```python
from build123d import *

# Parameters (mm, degrees)
FLOOR_2_DEPTH       = 5
SKETCH2_R           = 1.25
BOSS_EXTRUDE1_DEPTH = 5


with BuildPart() as part:
    # Sketch1 → Floor 2 (new body)
    with BuildSketch(Plane(origin=(0, 0, 0), x_dir=(1, 0, 0), z_dir=(0, 1, 0))):
        with BuildLine():
            Line((-46.9525, -71.4375), (46.9525, -71.4375))
            ThreePointArc((46.9525, -71.4375), (57.530817447, -67.055817447), (61.9125, -56.4775))
            Line((61.9125, -56.4775), (61.9125, 56.4775))
            ThreePointArc((61.9125, 56.4775), (57.530817447, 67.055817447), (46.9525, 71.4375))
            Line((46.9525, 71.4375), (-46.9525, 71.4375))
            ThreePointArc((-46.9525, 71.4375), (-57.530817447, 67.055817447), (-61.9125, 56.4775))
            Line((-61.9125, 56.4775), (-61.9125, -56.4775))
            ThreePointArc((-61.9125, -56.4775), (-57.530817447, -67.055817447), (-46.9525, -71.4375))
        make_face()
    extrude(amount=FLOOR_2_DEPTH)

    # Sketch2 → Boss-Extrude1 (add)
    # profile 1 of 4: a face of its own
    with BuildSketch(Plane(origin=(0, 5, 0), x_dir=(1, 0, 0), z_dir=(0, 1, 0))):
        Polygon((-56.370875673, -62.1125), (-57.814251346, -64.6125), (-56.370875673, -67.1125), (-53.484124327, -67.1125), (-52.040748654, -64.6125), (-53.484124327, -62.1125), align=None)
        with Locations(Location((-54.9275, -64.6125, 0), (0, 0, 270))):
            Circle(SKETCH2_R, mode=Mode.SUBTRACT)
    # profile 2 of 4: a face of its own
    with BuildSketch(Plane(origin=(0, 5, 0), x_dir=(1, 0, 0), z_dir=(0, 1, 0))):
        Polygon((56.055875673, -62.1125), (53.169124327, -62.1125), (51.725748654, -64.6125), (53.169124327, -67.1125), (56.055875673, -67.1125), (57.499251346, -64.6125), align=None)
        with Locations(Location((54.6125, -64.6125, 0), (0, 0, 270))):
            Circle(SKETCH2_R, mode=Mode.SUBTRACT)
    # profile 3 of 4: a face of its own
    with BuildSketch(Plane(origin=(0, 5, 0), x_dir=(1, 0, 0), z_dir=(0, 1, 0))):
        Polygon((-56.370875673, 66.4775), (-57.814251346, 63.9775), (-56.370875673, 61.4775), (-53.484124327, 61.4775), (-52.040748654, 63.9775), (-53.484124327, 66.4775), align=None)
        with Locations(Location((-54.9275, 63.9775, 0), (0, 0, 270))):
            Circle(SKETCH2_R, mode=Mode.SUBTRACT)
    # profile 4 of 4: a face of its own
    with BuildSketch(Plane(origin=(0, 5, 0), x_dir=(1, 0, 0), z_dir=(0, 1, 0))):
        Polygon((57.499251346, 63.9775), (56.055875673, 66.4775), (53.169124327, 66.4775), (51.725748654, 63.9775), (53.169124327, 61.4775), (56.055875673, 61.4775), align=None)
        with Locations(Location((54.6125, 63.9775, 0), (0, 0, 270))):
            Circle(SKETCH2_R, mode=Mode.SUBTRACT)
    extrude(amount=BOSS_EXTRUDE1_DEPTH)


solid = part.part
```
CAD build for the part. Positions are in the model's coordinates, mm. A direction names the side the tool comes from. Round coordinates to 2 decimals unless told otherwise and drop trailing zeros. Order: outer loops, then holes, each group sorted by start corner. A loop starts at its lowest first (then second) coordinate and runs counter-clockwise, first axis right, second up.
Item 1: Probe line 1 along Y through (x, z) = (9, 45); line 2 along X through (y, z) = (2.5, -57). List the from-to ranges inside material, lowest first.
Item 2: Pin check, flat tips, straight feed: pin 1 (2.5 mm diameter, centred on x = 54.5, y = 8.5, fed in from -Z); pin 2 (2.5 mm diameter, centred on x = 55, y = 7.5, fed in from +Z); pin 3 (2 mm diameter, centred on x = -54.93, z = 64.61, fed in from +Y). Stop position of each tip, or through.
Item 3: Saw through at B-B on z = 26. Write the cut outline in (x, y), then the cut area to 3 significant figures.
Item 4: Mould opens along Z. For faces 6 (the face through (-55, 7, -66.478)), 7 (the face through (-61.912, 2, -1)), 8 (the face through (57.414, 2.465, 67.171)), 9 (the face through (-55, 7, -61.478)) say: pulls with the +Z half, pulls with the -Z half, needs draft (parallel to the pull), parting line crosses it, or undercut.
Item 5: Tool access for faces 1 (the face through (-1, 2, 71.438)), 2 (the face through (55, 7, 67.112)), 3 (the face through (55, 7, -66.478)), 4 (the face through (-1, 5, -1)), 5 (the face through (-55, 7, 62.112)): list every direction of +Z, -Z, +X, -X, +Y, -Y with a clear straight run to the whole face (end or side of a thin tool).
Item 6: Saw through at A-A on y = 7.25. Write the cut outline in (x, z).
Item 7: Saw through at C-C on x = 39. Write the cut outline in (y, z).
Reported:
1. line 1: y = 0 to 5
1. line 2: x = -61.9 to 61.9
2. pin 1: stops at z = -66.48
2. pin 2: stops at z = 67.11
2. pin 3: stops at y = 5
3. outline: (-61.91, 0) - (61.91, 0) - (61.91, 5) - (-61.91, 5) - close
3. area: 619 mm2
4. face 6: pulls with the -Z half
4. face 7: needs draft
4. face 8: pulls with the +Z half
4. face 9: undercut
5. face 1: +Z, +X, -X, +Y, -Y
5. face 2: +Z, +X, -X, +Y
5. face 3: -Z, +X, -X, +Y
5. face 4: +Y
5. face 5: +X, -X, +Y
6. outline: (-57.81, -63.98) - (-56.37, -66.48) - (-53.48, -66.48) - (-52.04, -63.98) - (-53.48, -61.48) - (-56.37, -61.48) - close; (-57.81, 64.61) - (-56.37, 62.11) - (-53.48, 62.11) - (-52.04, 64.61) - (-53.48, 67.11) - (-56.37, 67.11) - close; (51.73, -63.98) - (53.17, -66.48) - (56.06, -66.48) - (57.5, -63.98) - (56.06, -61.48) - (53.17, -61.48) - close; (51.73, 64.61) - (53.17, 62.11) - (56.06, 62.11) - (57.5, 64.61) - (56.06, 67.11) - (53.17, 67.11) - close; hole circle Ø2.5 at (-54.93, -63.98); hole circle Ø2.5 at (-54.93, 64.61); hole circle Ø2.5 at (54.61, -63.98); hole circle Ø2.5 at (54.61, 64.61)
7. outline: (0, -71.44) - (5, -71.44) - (5, 71.44) - (0, 71.44) - close
